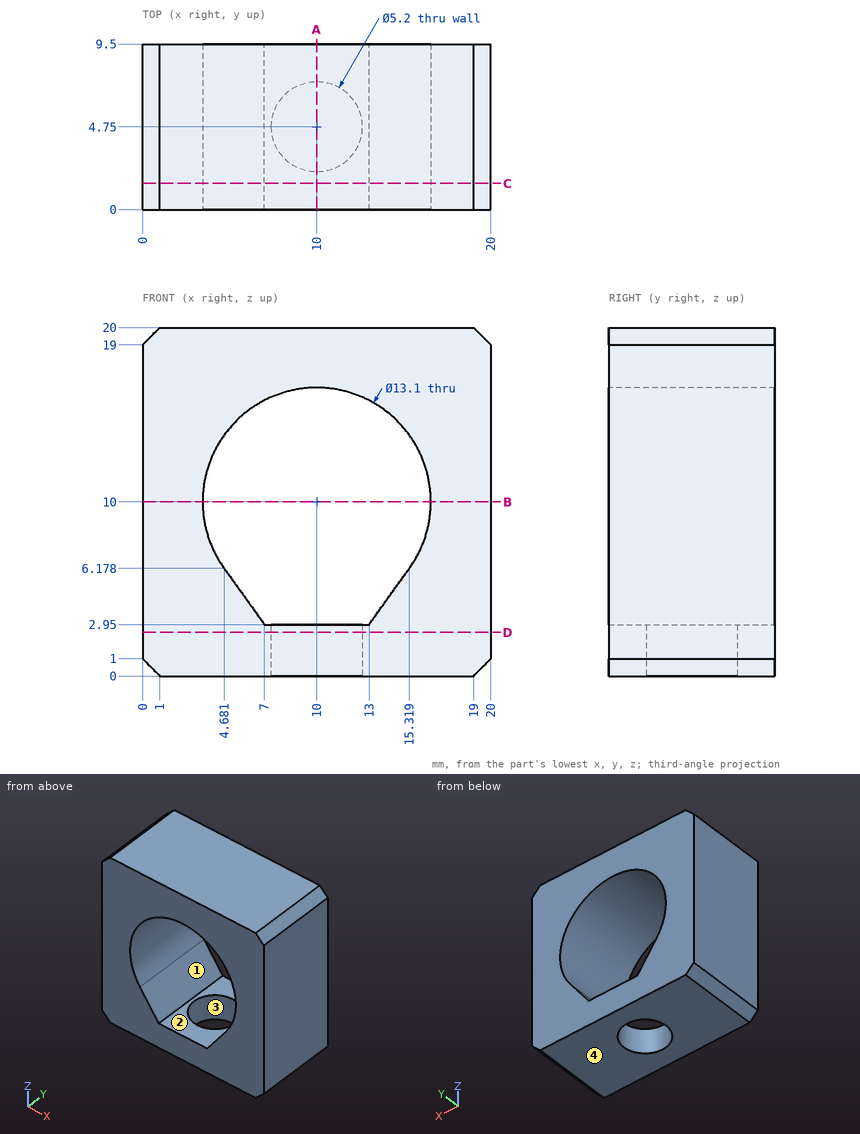
For this review, use the dimensioned drawing (mm, ordinates from the lowest corner) and the shaded views. Coordinates: 2 decimals unless noted, no trailing zeros. Loops run counter-clockwise (first coordinate to the right, second up) from the corner with the lowest first, then second, coordinate; pieces in that order, holes last. Notation, with made-up numbers: (51, 68.5) -> (108, 68.5) arc R20 cw to (108, 76.5) -> close; hole circle Ø11 at (-15, 67). An arc over 180 degrees is marked (long way). Return JSON: item names as keys, results as strings. Group by question number.
(1) Consider section D-D, the plane z = 2.5. Give the boundary of the cut face in (x, y), plus the area to 3 significant figures.
(2) Consider section A-A, the plane x = 10. Give the boundary of the cut face in (y, z).
(3) Mouldability with a two-part tool opening along Z and no side actions: class the marked faces 1, 2, 3 and 4 as pulls with the +Z half, pulls with the -Z half, needs draft (parallel to the pull), parting line crosses it, or undercut.
(4) Consider section B-B, the plane z = 10. Give the boundary of the cut face in (x, y).
(5) To check wall thickness, follow L1, parallel to Y at x = 10, z = 1.35; L2, parallel to X at y = 6.5, z = 10; L3, parallel to Z at x = 10, y = 4.5. State the ranges of each line that lie inside material, in increasing order.
(6) For pin 1 Ø6 at (x, z) = (8.5, 9.5) entering from -Y; pin 2 Ø4.5 at (x, y) = (10, 4.75) entering from -Z, all flat-tipped, find the tip position at first contact; note any pin that passes through.
(7) Consider section C-C, the plane y = 1.5. Give the boundary of the cut face in (x, z).
Results below:
{
 "1": {"outline": "(0, 0) -> (20, 0) -> (20, 9.5) -> (0, 9.5) -> close; hole circle Ø5.2 at (10, 4.75)", "area": "169 mm2"},
 "2": {"outline": "(0, 0) -> (2.15, 0) -> (2.15, 2.95) -> (0, 2.95) -> close; (0, 16.55) -> (9.5, 16.55) -> (9.5, 20) -> (0, 20) -> close; (7.35, 0) -> (9.5, 0) -> (9.5, 2.95) -> (7.35, 2.95) -> close"},
 "3": {"face 1": "undercut", "face 2": "undercut", "face 3": "needs draft", "face 4": "pulls with the -Z half"},
 "4": {"outline": "(0, 0) -> (3.45, 0) -> (3.45, 9.5) -> (0, 9.5) -> close; (16.55, 0) -> (20, 0) -> (20, 9.5) -> (16.55, 9.5) -> close"},
 "5": {"L1": "y = 0 to 2.15, 7.35 to 9.5", "L2": "x = 0 to 3.45, 16.55 to 20", "L3": "z = 16.55 to 20"},
 "6": {"pin 1": "passes through", "pin 2": "stops at z = 16.15"},
 "7": {"outline": "(0, 1) -> (1, 0) -> (19, 0) -> (20, 1) -> (20, 19) -> (19, 20) -> (1, 20) -> (0, 19) -> close; hole (4.68, 6.18) -> (7, 2.95) -> (13, 2.95) -> (15.32, 6.18) arc R6.55 ccw (long way) to start"}
}
